The listing builds one solid part. Answer for the finished solid, in the listing's coordinates (mm). A direction names the side the tool comes from. Coordinates: 2 decimals unless noted, no trailing zeros. Write each loop counter-clockwise with the first axis right and the second up, starting at its lowest first coordinate (ties: lowest second). Pieces come first, ordered by that corner, then holes. Notation, with made-up numbers: M 75.5,63 L 84.5,63 A31 cw 84.5,101 Z; hole C 20,88 d11. An arc over 180 degrees is marked long. Answer as a JSON object with one key per item and string values. Group by question number.
from build123d import *

# Parameters (mm, degrees)
SKETCH072_W            = 13.75
SKETCH072_H            = 13.75
PAD039_DEPTH           = 10
SKETCH073_W            = 20
SKETCH073_H            = 1
POCKET034_DEPTH        = 9
LINEARPATTERN001_COUNT = 6
LINEARPATTERN001_PITCH = 2


with BuildPart() as part:
    # Sketch072 → Pad039 (new body)
    with BuildSketch(Plane.XY):
        Rectangle(SKETCH072_W, SKETCH072_H)
    extrude(amount=PAD039_DEPTH)

    # Sketch073 → Pocket034 (cut)
    with BuildSketch(Plane(origin=(0, -5, 10), x_dir=(1, 0, 0), z_dir=(0, 0, 1))):
        Rectangle(SKETCH073_W, SKETCH073_H)
    pocket034 = extrude(amount=-POCKET034_DEPTH, mode=Mode.SUBTRACT)

    # LinearPattern001: Pocket034 ×6
    with Locations(*[(0, i * LINEARPATTERN001_PITCH, 0) for i in range(1, LINEARPATTERN001_COUNT)]):
        add(pocket034, mode=Mode.SUBTRACT)


solid = part.part
Item 1: A cutting plane is placed at B-B, the plane x = 4.5. Write down the section's boundary in (y, z) (3 decimals).
Item 2: A cutting plane is placed at A-A, the plane z = 1.75. Write down the section's boundary in (x, y) (3 decimals), and give its area (3 significant figures).
Item 3: A tool of negligible diameter and unlimited length cuts with its end or side. For faces 5 (the face through (0, -0.5, 6)), 6 (the face through (0, 0, 0)), from which of +Z, -Z, +X, -X, +Y, -Y can it reach the whole face along a straight path? Write none if from no direction.
Item 4: Consider L1, parallel to Z at x = 0.5, y = -2.75. Determine where the line is inside the solid, lowest interval first. Write a range as from..to.
Item 5: A cutting plane is placed at C-C, the plane y = -1.25. Write down the section's boundary in (x, z) (3 decimals).
Item 6: For a pull along Y with two mould halves and no side action, classify faces 1 (the face through (0, 6.875, 5)), 2 (the face through (0, 3, 1)), 3 (the face through (-6.875, 0, 5)), 4 (the face through (0, -4.5, 6)) as +Y half, -Y half, draft (parallel to the pull), parting line (faces both ways), or undercut.
Item 7: Flat-ended cylindrical pins translate along their axes: pin 1 Ø1.1 at (x, y) = (-1.5, -1) entering from +Z; pin 2 Ø0.8 at (x, y) = (1, 5) entering from +Z. Find the tip coordinate at first contact, or state that the pin passes through.
Answer:
{
 "1": {"outline": "M -6.875,0 L 6.875,0 L 6.875,10 L 5.5,10 L 5.5,1 L 4.5,1 L 4.5,10 L 3.5,10 L 3.5,1 L 2.5,1 L 2.5,10 L 1.5,10 L 1.5,1 L 0.5,1 L 0.5,10 L -0.5,10 L -0.5,1 L -1.5,1 L -1.5,10 L -2.5,10 L -2.5,1 L -3.5,1 L -3.5,10 L -4.5,10 L -4.5,1 L -5.5,1 L -5.5,10 L -6.875,10 Z"},
 "2": {"outline": "M -6.875,-6.875 L 6.875,-6.875 L 6.875,-5.5 L -6.875,-5.5 Z; M -6.875,-4.5 L 6.875,-4.5 L 6.875,-3.5 L -6.875,-3.5 Z; M -6.875,-2.5 L 6.875,-2.5 L 6.875,-1.5 L -6.875,-1.5 Z; M -6.875,-0.5 L 6.875,-0.5 L 6.875,0.5 L -6.875,0.5 Z; M -6.875,1.5 L 6.875,1.5 L 6.875,2.5 L -6.875,2.5 Z; M -6.875,3.5 L 6.875,3.5 L 6.875,4.5 L -6.875,4.5 Z; M -6.875,5.5 L 6.875,5.5 L 6.875,6.875 L -6.875,6.875 Z", "area": "107 mm2"},
 "3": {"face 5": "+Z, +X, -X", "face 6": "-Z, +X, -X, +Y, -Y"},
 "4": {"L1": "0..1"},
 "5": {"outline": "M -6.875,0 L 6.875,0 L 6.875,1 L -6.875,1 Z"},
 "6": {"face 1": "+Y half", "face 2": "undercut", "face 3": "draft", "face 4": "undercut"},
 "7": {"pin 1": "z = 10", "pin 2": "z = 1"}
}
